Answer from the drawing. Dimensions are ordinates in mm from the lowest x, y and z of the part. A direction names the side the tool comes from. Coordinates: 2 decimals unless noted, no trailing zeros. Loops run counter-clockwise (first coordinate to the right, second up) from the corner with the lowest first, then second, coordinate; pieces in that order, holes last. Notation, with made-up numbers: M 87.25,69.5 L 144.25,69.5 A21 ccw 144.25,93.5 Z; hole C 37.5,-21.5 d4. An arc over 180 degrees is marked long. One line per item, written item: value. Start each with the question number.
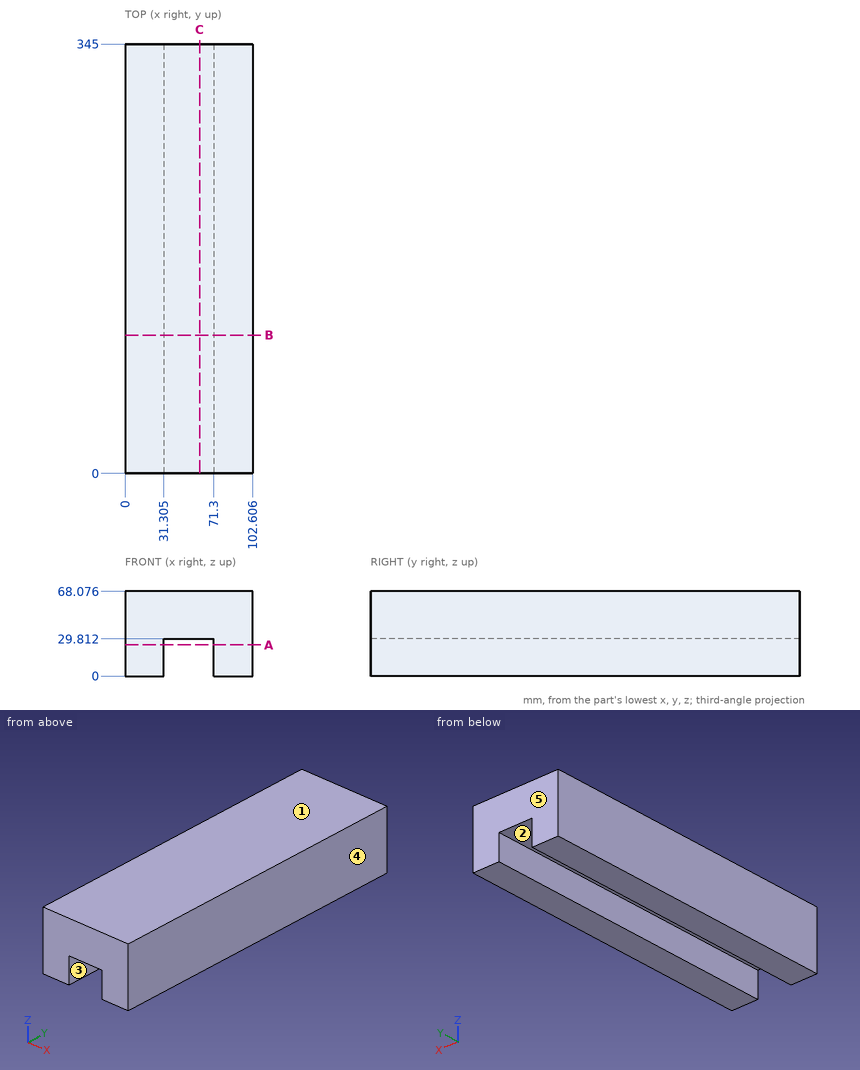
1) Consider line 1 along X through (y, z) = (76, 13.5) (1 decimal); line 2 along Z through (x, y) = (66, 330.5) (1 decimal). Determine where each line is inside the solid, lowest interval first.
2) Section C-C (x = 60) is taken. Determine the outline of the cut face in (y, z) (1 decimal), then the cut area to 3 significant figures.
3) Section A-A (z = 25) is taken. Determine the outline of the cut face in (x, y) (1 decimal).
4) A tool of negligible diameter and unlimited length cuts with its end or side. For the marked faces 1 and 2, from which of +Z, -Z, +X, -X, +Y, -Y can it reach the whole face along a straight path? Write none if from no direction.
5) Section B-B (y = 111) is taken. Determine the outline of the cut face in (x, z) (1 decimal), then the cut area to 3 significant figures.
6) For a pull along X with two mould halves and no side action, classify the marked faces 3, 4 and 5 as released by +X, released by -X, zero draft, split by the parting line, or undercut.
7) A flat-ended cylindrical pin translates along its axis: pin 1 (20 mm diameter, centred on x = 51.5, y = 255.5, fed in from -Z). Find the tip coordinate at first contact, or state that the pin passes through.
Results found:
1. line 1: x = 0 to 31.3, 71.3 to 102.6
1. line 2: z = 29.8 to 68.1
2. outline: M 0,29.8 L 345,29.8 L 345,68.1 L 0,68.1 Z
2. area: 13,200 mm²
3. outline: M 0,0 L 31.3,0 L 31.3,345 L 0,345 Z; M 71.3,0 L 102.6,0 L 102.6,345 L 71.3,345 Z
4. face 1: +Z, +X, -X, +Y, -Y
4. face 2: -Z, +Y, -Y
5. outline: M 0,0 L 31.3,0 L 31.3,29.8 L 71.3,29.8 L 71.3,0 L 102.6,0 L 102.6,68.1 L 0,68.1 Z
5. area: 5,790 mm²
6. face 3: undercut
6. face 4: released by +X
6. face 5: zero draft
7. pin 1: stops at z = 29.81
